Source: CAD feature listing. Evaluate the final solid. Frame: model axes, mm. A direction names the side the tool comes from. Give positions to 0.01 mm unless a question says otherwise; leave off trailing zeros. Write each loop counter-clockwise with the first axis right and the second up, starting at its lowest first coordinate (ties: lowest second). Pieces come first, ordered by that corner, then holes. Notation, with made-up numbers: (-8, -5) -> (41, -5) arc R12 cw to (41, 11) -> close; hole circle Ø4 at (-4.75, 74). An arc over 180 degrees is marked (long way). Answer as a JSON object with one key per item and string values. Group by question number.
Item 1: Section query A-A on z = 6. Return the cut outline in (x, y), plus the area to 3 significant figures.
Item 2: Pull-direction query (X, two-part tool) for faces 4 (the face through (0, -1, -15)), 5 (the face through (15, -1, 0)), 6 (the face through (-2.17, -40.28, -9.76)); classes: pulls with the +X half, pulls with the -X half, needs draft (parallel to the pull), parting line crosses it, or undercut.
Item 3: Access query for faces 1 (the face through (2.17, 40.28, -9.76)), 2 (the face through (0, -20, 0)), 3 (the face through (-15, -1, 0)). Directions: +Z, -Z, +X, -X, +Y, -Y. A direction counts if a zero-diameter tool reaches every point of the face in a straight line with its end or side. Return the directions, or none.
Item 4: Ray query, probe 1 along Z at (x, y) = (0, -40.5); probe 2 along Y at (x, z) = (-6.5, -2.75); probe 3 along X at (y, z) = (-31, -8). Return the intervals inside material, ascending. Write a range as from..to.
Item 5: First-contact query: pin 1 Ø1 at (x, z) = (3, 5.5) entering from -Y; pin 2 Ø12 at (x, z) = (0, 0) entering from +Y; pin 3 Ø16 at (x, z) = (2.5, 2.5) entering from +Y. Flat tips, straight axial feed; report the tip coordinate or a pass-through.
Item 6: Section query B-B on y = -30.5. Return the cut outline in (x, z), plus the area to 3 significant figures.
Item 7: Section query C-C on x = 0. Return the cut outline in (y, z), plus the area to 3 significant figures.
from build123d import *

# Parameters (mm, degrees)
F0_W     = 30
F0_H     = 30
F1_DEPTH = 60
F2_R     = 10
F3_DEPTH = 40
F4_R     = 10
F5_DEPTH = 40


with BuildPart() as f1:
    # F0 (on Front) → F1 (new body, symmetric)
    with BuildSketch(Plane.XZ):
        Rectangle(F0_W, F0_H)
    extrude(amount=F1_DEPTH, both=True)

    # F2 (on face) → F3 (cut)
    with BuildSketch(Plane(origin=(0, 60, 0), x_dir=(-1, 0, 0), z_dir=(0, 1, 0))):
        Circle(F2_R)
    extrude(amount=-F3_DEPTH, mode=Mode.SUBTRACT)

    # F4 (on face) → F5 (cut)
    with BuildSketch(Plane.XZ.offset(60)):
        Circle(F4_R)
    extrude(amount=-F5_DEPTH, mode=Mode.SUBTRACT)


solid = f1.part
Worked answers:
{
 "1": {"outline": "(-15, -60) -> (-8, -60) -> (-8, -20) -> (8, -20) -> (8, -60) -> (15, -60) -> (15, 60) -> (8, 60) -> (8, 20) -> (-8, 20) -> (-8, 60) -> (-15, 60) -> close", "area": "2,320 mm^2"},
 "2": {"face 4": "needs draft", "face 5": "pulls with the +X half", "face 6": "undercut"},
 "3": {"face 1": "+Y", "face 2": "-Y", "face 3": "+Z, -Z, -X, +Y, -Y"},
 "4": {"probe 1": "-15..-10, 10..15", "probe 2": "-20..20", "probe 3": "-15..-6, 6..15"},
 "5": {"pin 1": "y = -20", "pin 2": "y = 20", "pin 3": "y = 60"},
 "6": {"outline": "(-15, -15) -> (15, -15) -> (15, 15) -> (-15, 15) -> close; hole circle Ø20 at (0, 0)", "area": "586 mm^2"},
 "7": {"outline": "(-60, -15) -> (60, -15) -> (60, -10) -> (20, -10) -> (20, 10) -> (60, 10) -> (60, 15) -> (-60, 15) -> (-60, 10) -> (-20, 10) -> (-20, -10) -> (-60, -10) -> close", "area": "2,000 mm^2"}
}
